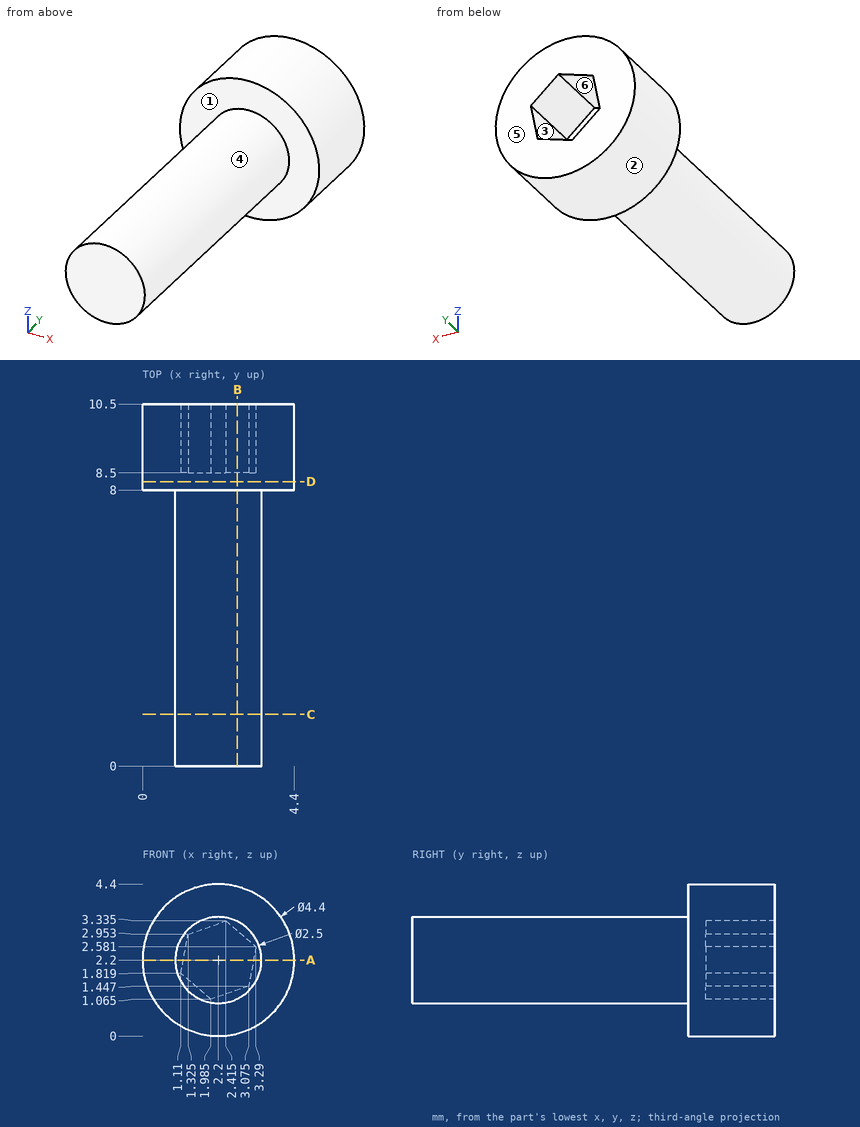
Answer from the drawing. Dimensions are ordinates in mm from the lowest x, y and z of the part. A direction names the side the tool comes from. Give positions to 0.01 mm unless a question says otherwise; leave off trailing zeros. Order: outer loops, then holes, each group sorted by start corner. A loop starts at its lowest first (then second) coordinate and runs counter-clockwise, first axis right, second up. Notation, with made-up numbers: (56, 54.25) -> (94, 54.25) arc R24 ccw to (94, 67.25) -> close; hole circle Ø2 at (42.25, 78). An arc over 180 degrees is marked (long way). One line per item, written item: value.
Item 1: Straight lines are drawn through the part: probe 1 along Y at (x, z) = (1.95, 2.6); probe 2 along Y at (x, z) = (1.6, 0.3); probe 3 along X at (y, z) = (9.75, 2.75) (1 decimal). For each, find the intervals that lie inside material, in ascending order.
Answer sheet:
probe 1: 0 to 8.5
probe 2: 8 to 10.5
probe 3: 0.1 to 1.3, 3.1 to 4.3
Item 2: Determine the mould class of the marked faces 4, 5 and 6 for opening direction X: released by +X, released by -X, zero draft, split by the parting line, or undercut.
Answer sheet:
face 4: split by the parting line
face 5: zero draft
face 6: undercut
Item 3: A tool of negligible diameter and unlimited length cuts with its end or side. For the marked faces 1, 2 and 3, from which of +Z, -Z, +X, -X, +Y, -Y can it reach the whole face along a straight path? Write none if from no direction.
Answer sheet:
face 1: -Y
face 2: +Y, -Y
face 3: +Y
Item 4: Find section B-B, the plane x = 2.75. Give the vertices of the cut face in (y, z), plus the area to 3 significant figures.
Answer sheet:
outline: (0, 1.08) -> (8, 1.08) -> (8, 0.07) -> (10.5, 0.07) -> (10.5, 1.33) -> (8.5, 1.33) -> (8.5, 3.05) -> (10.5, 3.05) -> (10.5, 4.33) -> (8, 4.33) -> (8, 3.32) -> (0, 3.32) -> close
area: 25.2 mm²
Item 5: Find section C-C, the plane y = 1.5. Give the vertices of the cut face in (x, z).
Answer sheet:
outline: circle Ø2.5 at (2.2, 2.2)
Item 6: Find section D-D, the plane y = 8.25. Give the vertices of the cut face in (x, z).
Answer sheet:
outline: circle Ø4.4 at (2.2, 2.2)
Item 7: Find section A-A, the plane z = 2.2. Give the vertices of the cut face in (x, y).
Answer sheet:
outline: (0, 8) -> (0.95, 8) -> (0.95, 0) -> (3.45, 0) -> (3.45, 8) -> (4.4, 8) -> (4.4, 10.5) -> (3.22, 10.5) -> (3.22, 8.5) -> (1.18, 8.5) -> (1.18, 10.5) -> (0, 10.5) -> close
